Read the model definition and answer for the solid it produces. Units are mm, in the model's axes. Face numbers are marked on the shaded views. A direction names the side the tool comes from. Round coordinates to 2 decimals unless told otherwise and drop trailing zeros. Loops run counter-clockwise (first coordinate to the right, second up) from the corner with the lowest first, then second, coordinate; pieces in that order, holes last. Notation, with made-up numbers: M -25.75,81 L 20.25,81 A34 ccw 20.25,113 Z; hole C 25.25,1.5 d9. An arc over 180 degrees is marked long. Answer as CSV lines item,"result".
```python
from build123d import *

# Parameters (mm, degrees)
BOSS_EXTRUDE1_DEPTH     = 8
CUT_EXTRUDE4_DEPTH      = 34
CUT_EXTRUDE4_DEPTH_BACK = 34
SKETCH2_R               = 3
SKETCH3_R               = 15
BOSS_EXTRUDE2_DEPTH     = 4
BOSS_EXTRUDE4_START     = -6
SKETCH3_5_R             = 15
SKETCH3_5_R_2           = 13.5
BOSS_EXTRUDE4_DEPTH     = 6
CUT_EXTRUDE5_DEPTH      = 8


# Read off the part's stored shape, not the designer's step: Cut-Extrude5
with BuildPart() as part:
    # Sketch1 → Boss-Extrude1 (new body)
    with BuildSketch(Plane.XY):
        Polygon((-25, -20), (25, -20), (25, 20), (15, 20), (15, 10), (-15, 10), (-15, 20), (-25, 20), align=None)
    extrude(amount=BOSS_EXTRUDE1_DEPTH)

    # Sketch2 → Cut-Extrude4 (cut, two sides: drawn at the far end of the back side and taken through both)
    with BuildSketch(Plane.XY.offset(-CUT_EXTRUDE4_DEPTH_BACK)):
        with Locations((-20, 15)):
            Circle(SKETCH2_R)
        with Locations((-20, -15)):
            Circle(SKETCH2_R)
        with Locations((20, -15)):
            Circle(SKETCH2_R)
        with Locations((20, 15)):
            Circle(SKETCH2_R)
    extrude(amount=CUT_EXTRUDE4_DEPTH + CUT_EXTRUDE4_DEPTH_BACK, mode=Mode.SUBTRACT)

    # Sketch3 → Boss-Extrude2 (add)
    with BuildSketch(Plane(origin=(0, 0, 0), x_dir=(1, 0, 0), z_dir=(0, 1, 0))):
        with BuildLine():
            Line((-16.5, -23), (-16.5, -7))
            Line((-16.5, -7), (16.5, -7))
            Line((16.5, -7), (16.5, -23))
            ThreePointArc((16.5, -23), (0, -39.5), (-16.5, -23))
        make_face()
        with Locations(Location((0, -23, 0), (0, 0, 90))):
            Circle(SKETCH3_R, mode=Mode.SUBTRACT)
    extrude(amount=BOSS_EXTRUDE2_DEPTH)

    # Sketch3<5> → Boss-Extrude4 (add)
    # profile 1 of 2: a face of its own
    with BuildSketch(Plane(origin=(0, 0, 0), x_dir=(1, 0, 0), z_dir=(0, 1, 0)).offset(BOSS_EXTRUDE4_START)):
        with BuildLine():
            Line((-16.5, -23), (-16.5, -7))
            Line((-16.5, -7), (16.5, -7))
            Line((16.5, -7), (16.5, -23))
            ThreePointArc((16.5, -23), (0, -39.5), (-16.5, -23))
        make_face()
        with Locations(Location((0, -23, 0), (0, 0, 90))):
            Circle(SKETCH3_5_R, mode=Mode.SUBTRACT)
    # profile 2 of 2: a face of its own
    with BuildSketch(Plane(origin=(0, 0, 0), x_dir=(1, 0, 0), z_dir=(0, 1, 0)).offset(BOSS_EXTRUDE4_START)):
        with Locations(Location((0, -23, 0), (0, 0, 90))):
            Circle(SKETCH3_5_R)
        with Locations(Location((0, -23, 0), (0, 0, 270))):
            Circle(SKETCH3_5_R_2, mode=Mode.SUBTRACT)
    extrude(amount=BOSS_EXTRUDE4_DEPTH)

    # Cut-Extrude5 outline → Cut-Extrude5 (cut)
    with BuildSketch(Plane.XY):
        with BuildLine():
            Line((25, 20), (22.360679775, 20))
            ThreePointArc((22.360679775, 20), (23.74188825, 18.339104186), (25, 16.583123952))
            Line((25, 16.583123952), (25, 20))
        make_face()
        with BuildLine():
            Line((-25, 20), (-25, 16.583123952))
            ThreePointArc((-25, 16.583123952), (-23.74188825, 18.339104186), (-22.360679775, 20))
            Line((-22.360679775, 20), (-25, 20))
        make_face()
        with BuildLine():
            Line((-25, -20), (-22.360679775, -20))
            ThreePointArc((-22.360679775, -20), (-23.74188825, -18.339104186), (-25, -16.583123952))
            Line((-25, -16.583123952), (-25, -20))
        make_face()
        with BuildLine():
            Line((25, -20), (25, -16.583123952))
            ThreePointArc((25, -16.583123952), (23.74188825, -18.339104186), (22.360679775, -20))
            Line((22.360679775, -20), (25, -20))
        make_face()
    extrude(amount=CUT_EXTRUDE5_DEPTH, mode=Mode.SUBTRACT)


solid = part.part
```
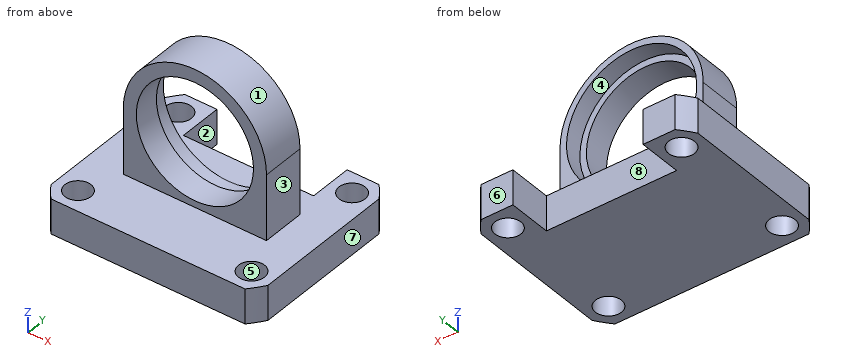
1) Straight lines are drawn through the part: line 1 (Y direction, x = -20, z = 4); line 2 (X direction, y = -15, z = 3.5); line 3 (X direction, y = 15, z = 5). For each, find the intervals that lie inside material, in ascending order.
Evaluation:
line 1,"y = -20 to -18, -12 to 12, 18 to 20"
line 2,"x = -25 to -23, -17 to 17, 23 to 25"
line 3,"x = -25 to -23, -17 to -15, 15 to 17, 23 to 25"
2) Find section A-A, the plane y = 15. Give the vertices of the cut face in (x, z), then the cut area to 3 significant figures.
Evaluation:
outline,"M -25,0 L -23,0 L -23,8 L -25,8 Z; M -17,0 L -15,0 L -15,8 L -17,8 Z; M 15,0 L 17,0 L 17,8 L 15,8 Z; M 23,0 L 25,0 L 25,8 L 23,8 Z"
area,"64.0 mm^2"
3) Find section C-C, the plane x = -20. Give the vertices of the cut face in (y, z).
Evaluation:
outline,"M -20,0 L -18,0 L -18,8 L -20,8 Z; M -12,0 L 12,0 L 12,8 L -12,8 Z; M 18,0 L 20,0 L 20,8 L 18,8 Z"
4) Find section B-B, the plane z = 4.5. Give the vertices of the cut face in (x, y), then the cut area to 3 significant figures.
Evaluation:
outline,"M -25,-16.58 A30 ccw -22.36,-20 L 22.36,-20 A30 ccw 25,-16.58 L 25,16.58 A30 ccw 22.36,20 L 15,20 L 15,10 L -15,10 L -15,20 L -22.36,20 A30 ccw -25,16.58 Z; hole C -20,-15 d6; hole C -20,15 d6; hole C 20,-15 d6; hole C 20,15 d6"
area,"1,570 mm^2"
5) A tool of negligible diameter and unlimited length cuts with its end or side. For the marked faces 1, 2, 3, 4 and 5, from which of +Z, -Z, +X, -X, +Y, -Y can it reach the whole face along a straight path? Write none if from no direction.
Evaluation:
face 1,"+Z, +Y, -Y"
face 2,"+Z, -Z, +Y"
face 3,"+Z, +X, +Y, -Y"
face 4,"+Y"
face 5,"+Z, -Z"
6) Find section D-D, the plane z = 30. Give the vertices of the cut face in (x, y).
Evaluation:
outline,"M -14.94,-6 L -11.54,-6 L -11.54,0 L -13.27,0 L -13.27,4 L -14.94,4 Z; M 11.54,-6 L 14.94,-6 L 14.94,4 L 13.27,4 L 13.27,0 L 11.54,0 Z"
7) Each of these flat-tipped pins is pushed along its axis until it touches: P1, Ø7, axis at x = -20, y = -15, coming from the +Z side; P2, Ø2.5, axis at y = 17, z = 3, coming from the +X side; P3, Ø8, axis at x = -13, y = 5.5, coming from the +Z side; P4, Ø9.5, axis at x = 3, z = 18, coming from the -Y side. Where does it stop, or does it pass through?
Evaluation:
P1,"stops at z = 8"
P2,"stops at x = 25"
P3,"stops at z = 36.63"
P4,"passes through"
8) Determine the mould class of the marked faces 6, 7 and 8 for opening direction X: released by +X, released by -X, zero draft, split by the parting line, or undercut.
Evaluation:
face 6,"zero draft"
face 7,"released by +X"
face 8,"undercut"
